Model file for the job. Use its own axes, mm. Round coordinates to 2 decimals unless told otherwise and drop trailing zeros. Loops run counter-clockwise (first coordinate to the right, second up) from the corner with the lowest first, then second, coordinate; pieces in that order, holes last. Notation, with made-up numbers: M 55.25,8.5 L 87.25,8.5 A26 ccw 87.25,25.5 Z; hole C 30.25,-23.75 d2. An arc over 180 degrees is marked long. Use a Markdown table: item, result. Add a question column.
Q1. Probe line 1 (X direction, y = 0.7, z = -28); line 2 (X direction, y = 1.25, z = 28); line 3 (X direction, y = 1.1, z = -39). List the from-to ranges inside material, lowest first. Write a range as from..to.
Q2. Cut at B-B (z = 28). Give the cut face in (x, y), plus the area to 3 significant figures.
Q3. Pin check, flat tips, straight feed: pin 1 (1.9 mm diameter, centred on x = -47, z = -28, fed in from +Y); pin 2 (0.6 mm diameter, centred on y = 1, z = -34.5, fed in from -X). Stop position of each tip, or through.
Q4. Cut at A-A (x = -47). Give the cut face in (y, z), plus the area to 3 significant figures.
Q5. Cut at C-C (z = -28). Give the cut face in (x, y).
Q6. Cut at D-D (x = 1). Give the cut face in (y, z), plus the area to 3 significant figures.
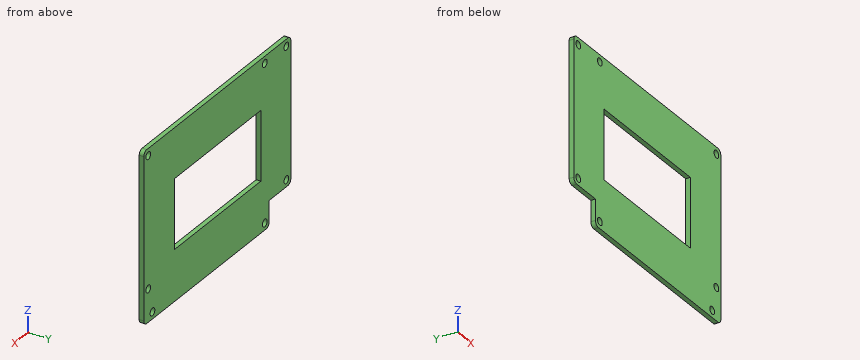
from build123d import *

# Parameters (mm, degrees)
SKETCH_1_R          = 1.6
EXTRUDE_1_DEPTH     = 2
CUT_EXTRUDE_1_REACH = 67.33
SKETCH_2_W          = 58.902173398
SKETCH_2_H          = 29.745647313


with BuildPart() as part:
    # 草图1 → 凸台-拉伸1 (new body)
    # profile 1 of 3: a face of its own
    with BuildSketch(Plane(origin=(0, 0, 0), x_dir=(1, 0, 0), z_dir=(0, 1, 0))):
        with BuildLine():
            Line((-35.3, -31), (48, -31))
            ThreePointArc((48, -31), (49.414213562, -30.414213562), (50, -29))
            Line((50, -29), (50, 29))
            ThreePointArc((50, 29), (49.414213562, 30.414213562), (48, 31))
            Line((48, 31), (-35.3, 31))
            Line((-35.3, 31), (-35.3, -31))
        make_face()
        with Locations(Location((-32.3, -28, 0), (0, 0, 270))):
            Circle(SKETCH_1_R, mode=Mode.SUBTRACT)
        with Locations(Location((47, -28, 0), (0, 0, 270))):
            Circle(SKETCH_1_R, mode=Mode.SUBTRACT)
        with Locations(Location((47, 28, 0), (0, 0, 270))):
            Circle(SKETCH_1_R, mode=Mode.SUBTRACT)
    # profile 2 of 3: a face of its own
    with BuildSketch(Plane(origin=(0, 0, 0), x_dir=(1, 0, 0), z_dir=(0, 1, 0))):
        with BuildLine():
            Line((-48, -31), (-35.3, -31))
            Line((-35.3, -31), (-35.3, 31))
            Line((-35.3, 31), (-48, 31))
            ThreePointArc((-48, 31), (-49.414213562, 30.414213562), (-50, 29))
            Line((-50, 29), (-50, -29))
            ThreePointArc((-50, -29), (-49.414213562, -30.414213562), (-48, -31))
        make_face()
        with Locations(Location((-47, -28, 0), (0, 0, 270))):
            Circle(SKETCH_1_R, mode=Mode.SUBTRACT)
        with Locations(Location((-47, 28, 0), (0, 0, 270))):
            Circle(SKETCH_1_R, mode=Mode.SUBTRACT)
    # profile 3 of 3: a face of its own
    with BuildSketch(Plane(origin=(0, 0, 0), x_dir=(1, 0, 0), z_dir=(0, 1, 0))):
        with BuildLine():
            Line((-35.3, 40), (-35.3, 31))
            Line((-35.3, 31), (48, 31))
            ThreePointArc((48, 31), (49.414213562, 30.414213562), (50, 29))
            Line((50, 29), (50, 40))
            ThreePointArc((50, 40), (49.414213562, 41.414213562), (48, 42))
            Line((48, 42), (-33.3, 42))
            ThreePointArc((-33.3, 42), (-34.714213562, 41.414213562), (-35.3, 40))
        make_face()
        with Locations(Location((-32.3, 39, 0), (0, 0, 270))):
            Circle(SKETCH_1_R, mode=Mode.SUBTRACT)
        with Locations(Location((44.144452232, 39, 0), (0, 0, 270))):
            Circle(SKETCH_1_R, mode=Mode.SUBTRACT)
    extrude(amount=EXTRUDE_1_DEPTH)

    # 草图2 → 切除-拉伸1 (cut, up to next)
    with BuildSketch(Plane(origin=(0, 2, 0), x_dir=(1, 0, 0), z_dir=(0, 1, 0)), mode=Mode.PRIVATE) as cut_extrude_1_sk1:
        with Locations((-0.141416386, 5.269425073)):
            Rectangle(SKETCH_2_W, SKETCH_2_H)
    cut_extrude_1_tool1 = extrude(cut_extrude_1_sk1.sketch, amount=-CUT_EXTRUDE_1_REACH, mode=Mode.PRIVATE) & part.part
    add(cut_extrude_1_tool1.solids().sort_by_distance((-0.141416, 2, -5.269425))[0], mode=Mode.SUBTRACT)


solid = part.part
Checked values:
| question | item | result |
|---|---|---|
| 1 | line 1 | x = -50..-48.6, -45.4..45.4, 48.6..50 |
| 1 | line 2 | x = -50..-48.6, -45.4..-33.9, -30.7..45.4, 48.6..50 |
| 1 | line 3 | x = -35.3..-33.9, -30.7..42.54, 45.74..50 |
| 2 | outline | M -50,0 L -48.6,0 L -48.6,2 L -50,2 Z; M -45.4,0 L -33.9,0 L -33.9,2 L -45.4,2 Z; M -30.7,0 L 45.4,0 L 45.4,2 L -30.7,2 Z; M 48.6,0 L 50,0 L 50,2 L 48.6,2 Z |
| 2 | area | 181 mm^2 |
| 3 | pin 1 | passes through |
| 3 | pin 2 | stops at x = -35.3 |
| 4 | outline | M 0,-31 L 2,-31 L 2,-29.6 L 0,-29.6 Z; M 0,-26.4 L 2,-26.4 L 2,26.4 L 0,26.4 Z; M 0,29.6 L 2,29.6 L 2,31 L 0,31 Z |
| 4 | area | 111 mm^2 |
| 5 | outline | M -50,0 L -48.6,0 L -48.6,2 L -50,2 Z; M -45.4,0 L 45.4,0 L 45.4,2 L -45.4,2 Z; M 48.6,0 L 50,0 L 50,2 L 48.6,2 Z |
| 6 | outline | M 0,-42 L 2,-42 L 2,-20.14 L 0,-20.14 Z; M 0,9.6 L 2,9.6 L 2,31 L 0,31 Z |
| 6 | area | 86.5 mm^2 |
